Could you check a few things on this model? Use its own coordinates, in mm. A direction names the side the tool comes from. Coordinates: 2 decimals unless noted, no trailing zeros. Loops run counter-clockwise (first coordinate to the right, second up) from the corner with the lowest first, then second, coordinate; pieces in that order, holes last. Notation, with made-up numbers: (-17, 33.25) -> (42, 33.25) arc R22 cw to (42, 49.25) -> close; hole circle Ø9 at (86, 59.25). An arc over 180 degrees is marked (long way). One line per question, with ' | ' between items.
```python
from build123d import *

# Parameters (mm, degrees)
F1_DEPTH = 65
F2_R     = 2
F3_R     = 2.548945
F3_R_2   = 2.548946
F3_R_3   = 2.548929
F3_R_4   = 4.347674
F3_R_5   = 3.974959
F4_DEPTH = 1.5
F5_R     = 1.75256
F5_R_2   = 1.752559
F6_DEPTH = 11.2
F7_DEPTH = 71


with BuildPart() as f1:
    # F0 (on Right) → F1 (new body)
    with BuildSketch(Plane.YZ):
        Polygon((0, -10.475962), (22.549306, -11.196655), (32.483309, 3.704351), (32.483309, 12.455739), (13.561399, 17.659265), (11.756126, 24.880352), (0, 17.659265), align=None)
    extrude(amount=F1_DEPTH)

    # F2
    f2_edges = [f1.edges().sort_by_distance(p)[0] for p in [
        (32.5, 32.483309, 3.704351),
        (32.5, 32.483309, 12.455739),
    ]]
    fillet(f2_edges, radius=F2_R)

    # F3 (on face) → F4 (join)
    with BuildSketch(Plane(origin=(0, 5.468337, 19.884858), x_dir=(1, 0, 0), z_dir=(0, 0.265157, 0.964205))):
        with Locations((50.906317, 21.071024)):
            Circle(F3_R)
        with Locations((44.022555, 20.437524)):
            Circle(F3_R)
        with Locations((44.650806, 13.906249)):
            Circle(F3_R_2)
        with Locations((51.875702, 14.267603)):
            Circle(F3_R)
        with Locations((22.165647, 13.906249)):
            Circle(F3_R)
        with Locations((15.557256, 13.906249)):
            Circle(F3_R)
        with Locations((15.832605, 21.071026)):
            Circle(F3_R)
        with Locations((22.716347, 20.437526)):
            Circle(F3_R_3)
        with Locations((5.347674, 17.519839)):
            Circle(F3_R_4)
        with Locations((60.025041, 18.603914)):
            Circle(F3_R_5)
    extrude(amount=F4_DEPTH)

    # F5 (on face) → F6 (join)
    with BuildSketch(Plane(origin=(0, 5.468337, 19.884858), x_dir=(1, 0, 0), z_dir=(0, 0.265157, 0.964205))):
        with Locations((60.025041, 18.603914)):
            Circle(F5_R)
        with Locations((5.347674, 17.519839)):
            Circle(F5_R_2)
    extrude(amount=F6_DEPTH)

    # F0 (on Right) → F7 (join)
    with BuildSketch(Plane.YZ):
        Polygon((0, -10.475962), (22.549306, -11.196655), (32.483309, 3.704351), (32.483309, 12.455739), (13.561399, 17.659265), (11.756126, 24.880352), (0, 17.659265), align=None)
    extrude(amount=F7_DEPTH)


solid = f1.part
```
Q1. For faces 4 (the face through (7.219, 21.886, 16.926)), 5 (the face through (43.99, 25.61, 15.9)), 6 (the face through (51.84, 19.657, 17.539)), 7 (the face through (35, 5.96, 21.32)), which set-ups out of +Z, -Z, +X, -X, +Y, -Y let a thin tool reach every point of the face, with its end or its side?
Values follow:
face 4: none | face 5: +Z, +Y | face 6: +Z, +X, +Y | face 7: +Z, +X, -X, -Y
Q2. Please list where these lines run through material, in increasing order: L1, parallel to X at y = 25, z = 16; L2, parallel to Z at x = 25.5, y = 9.5; L3, parallel to Y at x = 40, z = 2. Write a range as [from, to].
Values follow:
L1: x = [1.69, 9.01], [13.59, 18.08], [20.23, 25.2], [41.54, 46.51], [48.66, 53.15], [56.25, 63.8] | L2: z = [-10.78, 23.49] | L3: y = [0, 31.35]
Q3. Imagine slicing it at B-B on z = 22. Give the number of separate pieces and of enclosed holes in the cut face, plus the area to 3 significant figures.
Values follow:
separate pieces: 3 | enclosed holes: 0 | area: 404 mm2
Q4. Imagine slicing it at D-D on z = -2. Write out the boundary of the cut face in (x, y), plus the area to 3 significant figures.
Values follow:
outline: (0, 0) -> (71, 0) -> (71, 28.68) -> (0, 28.68) -> close | area: 2,040 mm2
Q5. We'd pull the mould along Y, two halves only. Please class faces 1 (the face through (0, 12, 3)), 2 (the face through (44.098, 16.674, 17.57)), 3 (the face through (35.003, 27.447, -3.85)): released by +Y, released by -Y, zero draft, split by the parting line, or undercut.
Values follow:
face 1: zero draft | face 2: undercut | face 3: released by +Y
Q6. Imagine slicing it at A-A on x = 30.5. Write out the boundary of the cut face in (y, z), plus the area to 3 significant figures.
Values follow:
outline: (0, -10.48) -> (22.55, -11.2) -> (32.48, 3.7) -> (32.48, 12.46) -> (13.56, 17.66) -> (11.76, 24.88) -> (0, 17.66) -> close | area: 855 mm2
Q7. Imagine slicing it at C-C on y = 8. Write out the boundary of the cut face in (x, z).
Values follow:
outline: (0, -10.73) -> (71, -10.73) -> (71, 22.57) -> (0, 22.57) -> close
